Design review of the part shown in the three views and the two pictorial views. Dimensions are in mm from the part's minimum x, y and z. Round coordinates to 2 decimals unless told otherwise and drop trailing zeros. Loops run counter-clockwise (first coordinate to the right, second up) from the corner with the lowest first, then second, coordinate; pieces in that order, holes last. Notation, with made-up numbers: (-33, 16.25) - (-2, 16.25) arc R19 ccw to (-2, 40.25) - close; hole circle Ø4 at (-9, 89). An arc over 180 degrees is marked (long way). Return JSON: item names as keys, results as strings. Group by question number.
(1) We need section B-B, the plane y = 30.5. Write out the cut boundary in (x, z), and give its area (3 significant figures).
(2) Wall thickness on L1, parallel to Y at x = 0.2, z = 18.5; L2, parallel to Z at x = 0.85, y = 8; L3, parallel to Z at x = 1.65, y = 29: over which ranges is each line inside the solid? List them lowest first. Write a range as [from, to].
(3) We need section A-A, the plane x = 0.75. Write out the cut boundary in (y, z).
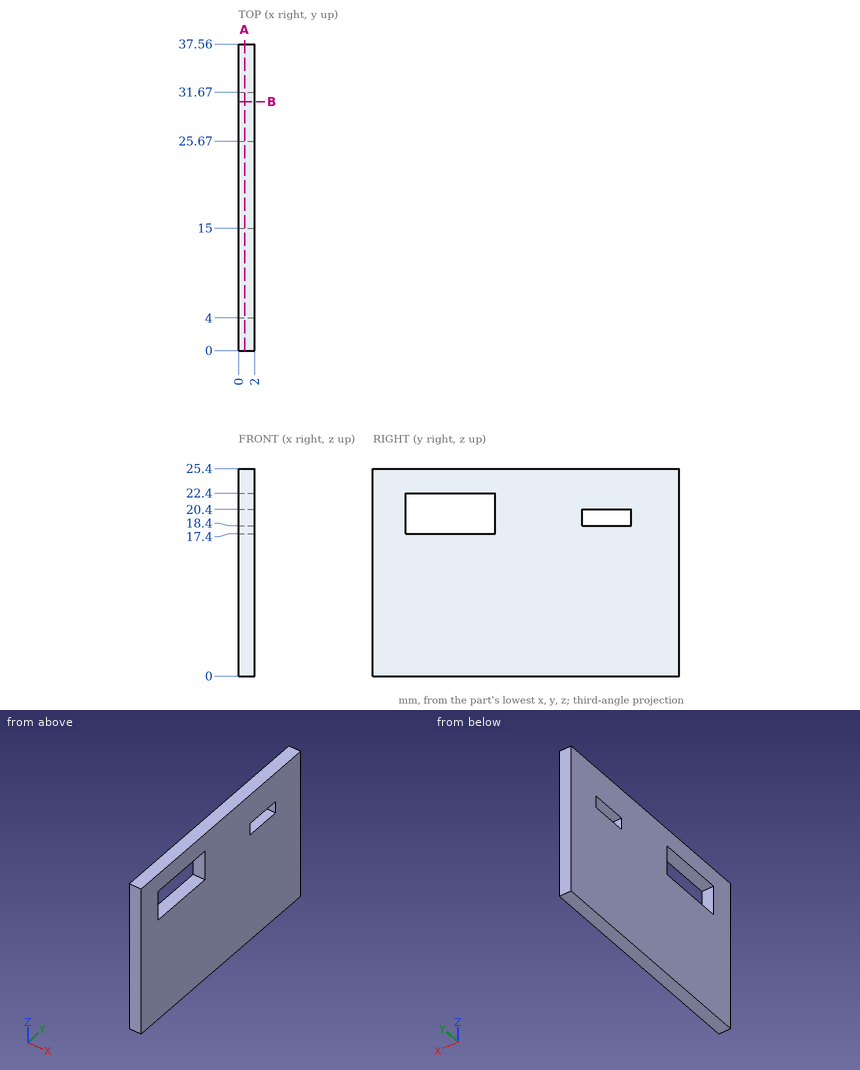
Solutions:
{
 "1": {"outline": "(0, 0) - (2, 0) - (2, 18.4) - (0, 18.4) - close; (0, 20.4) - (2, 20.4) - (2, 25.4) - (0, 25.4) - close", "area": "46.8 mm^2"},
 "2": {"L1": "[0, 4], [15, 25.67], [31.67, 37.56]", "L2": "[0, 17.4], [22.4, 25.4]", "L3": "[0, 18.4], [20.4, 25.4]"},
 "3": {"outline": "(0, 0) - (37.56, 0) - (37.56, 25.4) - (0, 25.4) - close; hole (4, 17.4) - (15, 17.4) - (15, 22.4) - (4, 22.4) - close; hole (25.67, 18.4) - (31.67, 18.4) - (31.67, 20.4) - (25.67, 20.4) - close"}
}
